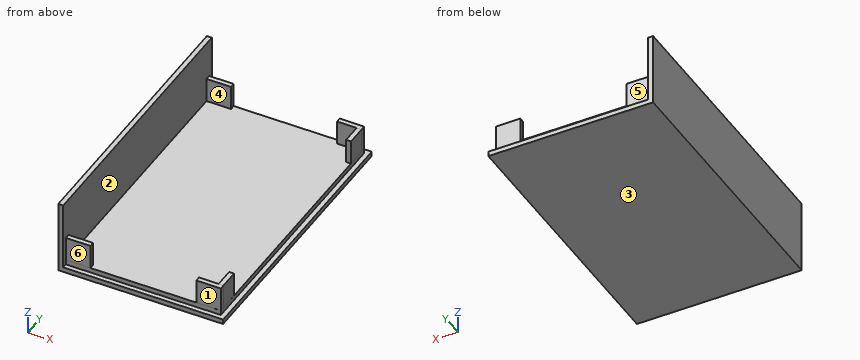
from build123d import *

# Parameters (mm, degrees)
SKETCH_W     = 67.25
SKETCH_H     = 112.8
PAD_DEPTH    = 30
THICKNESS_T  = -2
SKETCH001_W  = 63.25
SKETCH001_H  = 108.800063
PAD001_DEPTH = 2
SKETCH002_W  = 10
SKETCH002_H  = 2
PAD002_DEPTH = 10
SKETCH003_W  = 10
SKETCH003_H  = 2
PAD003_DEPTH = 10
SKETCH004_W  = 2
SKETCH004_H  = 8
PAD004_DEPTH = 10
SKETCH005_W  = 10
SKETCH005_H  = 2
PAD005_DEPTH = 10
SKETCH006_W  = 2
SKETCH006_H  = 8
PAD006_DEPTH = 10
SKETCH007_W  = 10
SKETCH007_H  = 2
PAD007_DEPTH = 10


with BuildPart() as part:
    # Sketch → Pad (new body)
    with BuildSketch(Plane.XY):
        with Locations((33.625, 56.4)):
            Rectangle(SKETCH_W, SKETCH_H)
    extrude(amount=PAD_DEPTH)

    # Thickness
    thickness_openings = [part.faces().sort_by_distance(p)[0] for p in [
        (67.25, 56.4, 15),
        (33.625, 0, 15),
        (33.625, 56.4, 30),
        (33.625, 112.8, 15),
    ]]
    offset(amount=THICKNESS_T, openings=thickness_openings)

    # Sketch001 (on Face8 of Thickness) → Pad001 (join)
    with BuildSketch(Plane.XY.offset(2)):
        with Locations((33.630087, 56.399667)):
            Rectangle(SKETCH001_W, SKETCH001_H)
    extrude(amount=PAD001_DEPTH)

    # Sketch002 (on Face13 of Pad001) → Pad002 (join)
    with BuildSketch(Plane.XY.offset(4)):
        with Locations((7.005123, 2.998829)):
            Rectangle(SKETCH002_W, SKETCH002_H)
    extrude(amount=PAD002_DEPTH)

    # Sketch003 (on Face13 of Pad002) → Pad003 (join)
    with BuildSketch(Plane.XY.offset(4)):
        with Locations((60.25087, 3.005487)):
            Rectangle(SKETCH003_W, SKETCH003_H)
    extrude(amount=PAD003_DEPTH)

    # Sketch004 (on Face13 of Pad003) → Pad004 (join)
    with BuildSketch(Plane.XY.offset(4)):
        with Locations((64.250015, 8.00565)):
            Rectangle(SKETCH004_W, SKETCH004_H)
    extrude(amount=PAD004_DEPTH)

    # Sketch005 (on Face13 of Pad004) → Pad005 (join)
    with BuildSketch(Plane.XY.offset(4)):
        with Locations((60.255219, 109.799278)):
            Rectangle(SKETCH005_W, SKETCH005_H)
    extrude(amount=PAD005_DEPTH)

    # Sketch006 (on Face13 of Pad005) → Pad006 (join)
    with BuildSketch(Plane.XY.offset(4)):
        with Locations((64.253967, 104.795769)):
            Rectangle(SKETCH006_W, SKETCH006_H)
    extrude(amount=PAD006_DEPTH)

    # Sketch007 (on Face13 of Pad006) → Pad007 (join)
    with BuildSketch(Plane.XY.offset(4)):
        with Locations((7.006138, 109.796768)):
            Rectangle(SKETCH007_W, SKETCH007_H)
    extrude(amount=PAD007_DEPTH)


solid = part.part
Design review of the part built by this model. Coordinates are the model's own, in mm. Face numbers are marked on the shaded views. A direction names the side the tool comes from. Give positions to 0.01 mm unless a question says otherwise; leave off trailing zeros. Loops run counter-clockwise (first coordinate to the right, second up) from the corner with the lowest first, then second, coordinate; pieces in that order, holes last. Notation, with made-up numbers: (-9, -40) - (-3, -40) arc R18 cw to (-3, -15) - close; hole circle Ø11 at (81, -38). An arc over 180 degrees is marked (long way). Use CSV: the item, a comma, the result in double quotes. Start each with the question number.
1. Draft analysis for pull direction Y (two halves, no side actions). For the marked faces 1, 2 and 3, state which applies: released by +Y, released by -Y, zero draft, split by the parting line, or undercut.
2. Wall thickness on L1, parallel to Y at x = 61, z = 4.5; L2, parallel to X at y = 63.5, z = 24; L3, parallel to Z at x = 33, y = 27: over which ranges is each line inside the solid? List them lowest first.
3. Machinability: for the marked faces 4, 5 and 6, which of the approach directions +Z, -Z, +X, -X, +Y, -Y give a long, thin tool a straight path to every point of the face, cutting with its end or side? Answer none if there is none.
4. Insertion check: P1, Ø1.6, axis at y = 109.5, z = 8.5, coming from the +X side; P2, Ø1.6, axis at x = 32, z = 3, coming from the -Y side; P3, Ø12, axis at x = 22, y = 51, coming from the +Z side. Each pin has a flat end and moves straight along its axis. Give the tip position at first contact, or say it passes through.
5. Add section A-A (z = 10.75). State the section outline as (x, y) points, plus the area to 3 significant figures.
6. Add section D-D (z = 16). State the section outline as (x, y) points, plus the area to 3 significant figures.
Results found:
1,face 1,"released by -Y"
1,face 2,"undercut"
1,face 3,"zero draft"
2,L1,"y = 2.01 to 4.01, 108.8 to 110.8"
2,L2,"x = 0 to 2"
2,L3,"z = 0 to 4"
3,face 4,"+Z"
3,face 5,"+Z, +X, +Y"
3,face 6,"+Z, +X, -Y"
4,P1,"stops at x = 65.26"
4,P2,"stops at y = 2"
4,P3,"stops at z = 4"
5,outline,"(0, 0) - (2, 0) - (2, 112.8) - (0, 112.8) - close; (2.01, 2) - (12.01, 2) - (12.01, 4) - (2.01, 4) - close; (2.01, 108.8) - (12.01, 108.8) - (12.01, 110.8) - (2.01, 110.8) - close; (55.25, 2.01) - (65.25, 2.01) - (65.25, 4.01) - (55.25, 4.01) - close; (55.26, 108.8) - (65.26, 108.8) - (65.26, 110.8) - (55.26, 110.8) - close; (63.25, 4.01) - (65.25, 4.01) - (65.25, 12.01) - (63.25, 12.01) - close; (63.25, 100.8) - (65.25, 100.8) - (65.25, 108.8) - (63.25, 108.8) - close"
5,area,"338 mm²"
6,outline,"(0, 0) - (2, 0) - (2, 112.8) - (0, 112.8) - close"
6,area,"226 mm²"
